For this review, take the finished solid that the model builds, in its own axes (mm). A direction names the side the tool comes from. Round coordinates to 2 decimals unless told otherwise and drop trailing zeros. Write each question's results on one line, items separated by ' | '. Start each with the question number.
Item 1: Add section A-A (x = 0.55). Count the separate pieces of the cut face and the enclosed holes in it, plus the area to 3 significant figures.
Item 2: To check wall thickness, follow line 1 along Z through (x, y) = (0.75, 490); line 2 along Z through (x, y) = (0.65, 432); line 3 along Y through (x, z) = (1.2, -342). State the ranges of each line that lie inside material, in increasing order.
Item 3: Clearance check with flat-ended pins moving along their axes: pin 1 (5.5 mm diameter, centred on y = 288, z = -10, fed in from +X); pin 2 (0.7 mm diameter, centred on x = 1, z = -385.5, fed in from +Y). State where each tip first meets the part, or that it passes through.
Item 4: Tool access review of faces 1 (the flat face through (1, 270, -350)), 2 (the flat face through (1, 50, -60)), 3 (the flat face through (1, 270, -60)): name each direction out of +Z, -Z, +X, -X, +Y, -Y from which nothing blocks a thin tool from reaching the whole face with its end or side.
Item 5: The part is to be moulded in two halves that separate along Y. For faces 4 (the flat face through (0, 254, -202)), 5 (the flat face through (1, 190, -350)), 6 (the flat face through (1, 50, -350)), say which applies: +Y half, -Y half, draft (parallel to the pull), parting line (faces both ways), or undercut.
from build123d import *

# Parameters (mm, degrees)
BOSS_EXTRUDE1_DEPTH = 1.31064
SKETCH2_R           = 3.1
CUT_EXTRUDE1_DEPTH  = 10


with BuildPart() as part:
    # Sketch1 → Boss-Extrude1 (new body)
    with BuildSketch(Plane(origin=(0, 0, 0), x_dir=(0, 0, -1), z_dir=(1, 0, 0))):
        Polygon((0, 440), (0, 280), (40, 280), (80, 260), (80, 200), (40, 180), (0, 180), (0, 80), (40, 80), (80, 20), (80, 0), (330, 0), (330, 20), (370, 80), (410, 80), (410, 180), (370, 180), (330, 200), (330, 260), (370, 280), (410, 280), (410, 440), (350, 440), (350, 500), (60, 500), (60, 440), align=None)
    extrude(amount=BOSS_EXTRUDE1_DEPTH)

    # Sketch2 → Cut-Extrude1 (cut)
    with BuildSketch(Plane(origin=(1.31064, 0, 0), x_dir=(0, 0, -1), z_dir=(1, 0, 0))):
        with Locations((10, 432)):
            Circle(SKETCH2_R)
        with Locations((10, 288)):
            Circle(SKETCH2_R)
        with Locations((10, 172)):
            Circle(SKETCH2_R)
        with Locations((10, 88)):
            Circle(SKETCH2_R)
        with Locations((88, 10)):
            Circle(SKETCH2_R)
        with Locations((68, 490)):
            Circle(SKETCH2_R)
        with Locations((322, 10)):
            Circle(SKETCH2_R)
        with Locations((400, 88)):
            Circle(SKETCH2_R)
        with Locations((400, 172)):
            Circle(SKETCH2_R)
        with Locations((400, 288)):
            Circle(SKETCH2_R)
        with Locations((400, 432)):
            Circle(SKETCH2_R)
        with Locations((342, 490)):
            Circle(SKETCH2_R)
    extrude(amount=-CUT_EXTRUDE1_DEPTH, mode=Mode.SUBTRACT)


solid = part.part
Responses:
1) separate pieces: 1 | enclosed holes: 12 | area: 173,000 mm^2
2) line 1: z = -350 to -345.1, -338.9 to -71.1, -64.9 to -60 | line 2: z = -410 to -403.1, -396.9 to -13.1, -6.9 to 0 | line 3: y = 38 to 194, 266 to 486.9, 493.1 to 500
3) pin 1: passes through | pin 2: stops at y = 440
4) face 1: -Z, +X, -X | face 2: +Z, +X, -X, -Y | face 3: +Z, +X, -X
5) face 4: draft | face 5: undercut | face 6: -Y half
